Input: part model. Units: mm. Frame: model coordinates. Face numbers are marked on the shaded views. A direction names the side the tool comes from. Give positions to 0.01 mm unless a question says otherwise; leave off trailing zeros. Loops run counter-clockwise (first coordinate to the right, second up) from the corner with the lowest first, then second, coordinate; pieces in that order, holes last. Notation, with made-up numbers: (43.25, 35) - (66.25, 35) arc R20 cw to (66.25, 42) - close; hole circle Ø10 at (74.5, 43). An arc over 180 degrees is marked (long way). Answer as a JSON object with one key per item and string values. Group by question number.
(1) Material intervals for L1, parallel to Y at x = 1, z = -7.25; L2, parallel to X at y = -13.25, z = -8; L3, parallel to Y at x = -2.5, z = -10.75, sorted ascending.
(2) Mould query, pull axis X, two halves, no side actions, for the marked faces 3, 4, 5 and 6. Classes: +X half, -X half, draft (parallel to the pull), parting line (faces both ways), or undercut.
(3) Section query B-B (y = -5). Return loops of the section in (x, z), plus the area to 3 significant figures.
(4) Pin query (flat end, axial travel): P1, Ø5, axis at y = -7, z = -6, coming from the -X side. Return the tip coordinate at first contact, or that it passes through.
(5) Access query for the marked faces 1 and 2. Directions: +Z, -Z, +X, -X, +Y, -Y. A direction counts if a zero-diameter tool reaches every point of the face in a straight line with its end or side. Return the directions, or none.
(6) Section query A-A (x = 0.25). Return loops of the section in (y, z), plus the area to 3 significant figures.
```python
from build123d import *

# Parameters (mm, degrees)
SKETCH1_W           = 11.176
SKETCH1_H           = 10.16
BOSS_EXTRUDE1_DEPTH = 3.048
SKETCH2_W           = 3.048
SKETCH2_H           = 10.16
BOSS_EXTRUDE2_DEPTH = 19.0815
SKETCH3_W           = 10.16
SKETCH3_H           = 3.048
BOSS_EXTRUDE3_DEPTH = 8.128
SKETCH4_W           = 3.048
SKETCH4_H           = 10.16
BOSS_EXTRUDE4_DEPTH = 1.27
BOSS_EXTRUDE4_TAPER = 45


with BuildPart() as part:
    # Sketch1 → Boss-Extrude1 (new body)
    with BuildSketch(Plane.XZ.offset(13.5255)):
        with Locations((2.54, -8.349079223)):
            Rectangle(SKETCH1_W, SKETCH1_H)
    extrude(amount=BOSS_EXTRUDE1_DEPTH)

    # Sketch2 → Boss-Extrude2 (add)
    with BuildSketch(Plane(origin=(0, -13.5255, 0), x_dir=(1, 0, 0), z_dir=(0, 1, 0))):
        with Locations((6.604, 8.349079223)):
            Rectangle(SKETCH2_W, SKETCH2_H)
    extrude(amount=BOSS_EXTRUDE2_DEPTH)

    # Sketch3 → Boss-Extrude3 (add)
    with BuildSketch(Plane.ZY.offset(-5.08)):
        with Locations((-8.349079223, 4.032)):
            Rectangle(SKETCH3_W, SKETCH3_H)
    extrude(amount=BOSS_EXTRUDE3_DEPTH)

    # Sketch4 → Boss-Extrude4 (add)
    with BuildSketch(Plane.XZ.offset(-2.508)):
        with Locations((-1.524, -8.349079223)):
            Rectangle(SKETCH4_W, SKETCH4_H)
    extrude(amount=BOSS_EXTRUDE4_DEPTH, taper=BOSS_EXTRUDE4_TAPER)


solid = part.part
```
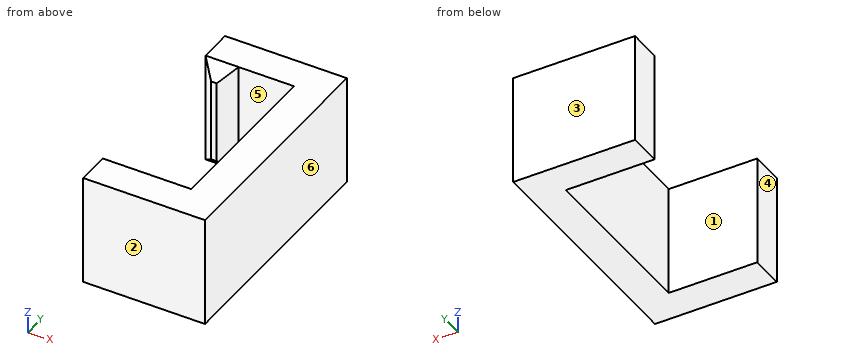
Recorded:
{
 "1": {"L1": "y = -16.57 to -13.53, 2.51 to 5.56", "L2": "x = 5.08 to 8.13", "L3": "y = -16.57 to -13.53, 1.96 to 5.56"},
 "2": {"face 3": "draft", "face 4": "-X half", "face 5": "undercut", "face 6": "+X half"},
 "3": {"outline": "(5.08, -13.43) - (8.13, -13.43) - (8.13, -3.27) - (5.08, -3.27) - close", "area": "31.0 mm^2"},
 "4": {"P1": "stops at x = 5.08"},
 "5": {"face 1": "+Z, -Z, -X", "face 2": "+Z, -Z, +X, -X, -Y"},
 "6": {"outline": "(-16.57, -13.43) - (-13.53, -13.43) - (-13.53, -3.27) - (-16.57, -3.27) - close; (2.51, -13.43) - (5.56, -13.43) - (5.56, -3.27) - (2.51, -3.27) - close", "area": "61.9 mm^2"}
}
